```python
from build123d import *

# Parameters (mm, degrees)
SKETCH_W        = 40
SKETCH_H        = 26
PAD_DEPTH       = 6
SKETCH001_W     = 46
SKETCH001_H     = 21
POCKET_DEPTH    = 3.5
SKETCH002_R     = 1.7
POCKET001_DEPTH = 2.5
SKETCH003_W     = 20
SKETCH003_H     = 20
PAD001_DEPTH    = 15
SKETCH004_R     = 6.2
POCKET002_DEPTH = 15
FILLET_R        = 5


with BuildPart() as part:
    # Sketch → Pad (new body)
    with BuildSketch(Plane.XY):
        Rectangle(SKETCH_W, SKETCH_H)
    extrude(amount=PAD_DEPTH)

    # Sketch001 (on Face5 of Pad) → Pocket (cut)
    with BuildSketch(Plane(origin=(0, 0, 0), x_dir=(1, 0, 0), z_dir=(0, 0, -1))):
        Rectangle(SKETCH001_W, SKETCH001_H)
    extrude(amount=-POCKET_DEPTH, mode=Mode.SUBTRACT)

    # Sketch002 (on Face5 of Pocket) → Pocket001 (cut)
    with BuildSketch(Plane.XY.offset(6)):
        with Locations((-15, 5)):
            Circle(SKETCH002_R)
        with Locations((15, 5)):
            Circle(SKETCH002_R)
        with Locations((15, -5)):
            Circle(SKETCH002_R)
        with Locations((-15, -5)):
            Circle(SKETCH002_R)
    extrude(amount=-POCKET001_DEPTH, mode=Mode.SUBTRACT)

    # Sketch003 (on Face5 of Pocket001) → Pad001 (join)
    with BuildSketch(Plane.XY.offset(6)):
        Rectangle(SKETCH003_W, SKETCH003_H)
    extrude(amount=PAD001_DEPTH)

    # Sketch004 (on Face19 of Pad001) → Pocket002 (cut)
    with BuildSketch(Plane.XY.offset(21)):
        Circle(SKETCH004_R)
    extrude(amount=-POCKET002_DEPTH, mode=Mode.SUBTRACT)

    # Fillet
    fillet_edges = [part.edges().sort_by_distance(p)[0] for p in [
        (-10, -10, 13.5),
        (-10, 10, 13.5),
        (10, -10, 13.5),
        (10, 10, 13.5),
    ]]
    fillet(fillet_edges, radius=FILLET_R)


solid = part.part
```
Verification items for the finished model (mm, model axes). A direction names the side the tool comes from. Give positions to 0.01 mm unless a question says otherwise; leave off trailing zeros. Loops run counter-clockwise (first coordinate to the right, second up) from the corner with the lowest first, then second, coordinate; pieces in that order, holes last.
1. Section check B-B, the plane x = 15. Enter the section's corners in (y, z).
2. Section check A-A, the plane z = 19. Enter the section's corners in (x, y), then the cut area to 3 significant figures.
3. Mould release check, pull along X, two halves, no side actions. Record for faces 4 (the flat face through (20, 0, 4)), 5 (the flat face through (0, 0, 6)), 6 (the flat face through (-20, 0, 4)), 7 (the flat face through (0, -10, 13)): released by +X, released by -X, zero draft, split by the parting line, or undercut.
4. Thickness scan on line 1 (Y direction, x = 15, z = 4.4); line 2 (Y direction, x = 18.5, z = 2); line 3 (Z direction, x = 17.5, y = -6.75). Record the ranges inside material, lowest first.
5. Section check C-C, the plane y = 4.5. Enter the section's corners in (x, z), then the cut area to 3 significant figures.
6. Set-up check for faces 1 (the flat face through (0, 0, 3.5)), 2 (the flat face through (-10, 0, 13)), 3 (the flat face through (0, 10, 13)): record each of +Z, -Z, +X, -X, +Y, -Y from which the full face is reachable in a straight line by a thin tool's end or side.
7. Go/stop test with flat-tipped pins: pin 1 Ø5 at (x, z) = (-1, 13.5) entering from +Y; pin 2 Ø3.5 at (x, y) = (-2, 2.5) entering from +Z; pin 3 Ø10.5 at (x, y) = (4.5, 3) entering from -Z; pin 4 Ø2.5 at (x, y) = (-15, 5) entering from -Z. Record where each tip stops, or that it passes through.
8. Section check D-D, the plane z = 1.5. Enter the section's corners in (x, y), then the cut area to 3 significant figures.
Geometry says:
1. outline: (-13, 0) - (-10.5, 0) - (-10.5, 3.5) - (-6.7, 3.5) - (-6.7, 6) - (-13, 6) - close; (-3.3, 3.5) - (3.3, 3.5) - (3.3, 6) - (-3.3, 6) - close; (6.7, 3.5) - (10.5, 3.5) - (10.5, 0) - (13, 0) - (13, 6) - (6.7, 6) - close
2. outline: (-10, -5) arc R5 ccw to (-5, -10) - (5, -10) arc R5 ccw to (10, -5) - (10, 5) arc R5 ccw to (5, 10) - (-5, 10) arc R5 ccw to (-10, 5) - close; hole circle Ø12.4 at (0, 0)
2. area: 258 mm2
3. face 4: released by +X
3. face 5: undercut
3. face 6: released by -X
3. face 7: zero draft
4. line 1: y = -13 to -6.7, -3.3 to 3.3, 6.7 to 13
4. line 2: y = -13 to -10.5, 10.5 to 13
4. line 3: z = 3.5 to 6
5. outline: (-20, 3.5) - (-16.62, 3.5) - (-16.62, 6) - (-20, 6) - close; (-13.38, 3.5) - (13.38, 3.5) - (13.38, 6) - (10, 6) - (10, 21) - (4.26, 21) - (4.26, 6) - (-4.26, 6) - (-4.26, 21) - (-10, 21) - (-10, 6) - (-13.38, 6) - close; (16.62, 3.5) - (20, 3.5) - (20, 6) - (16.62, 6) - close
5. area: 256 mm2
6. face 1: -Z, +X, -X
6. face 2: +Z, -X, +Y, -Y
6. face 3: +Z, +X, -X, +Y
7. pin 1: stops at y = 10
7. pin 2: stops at z = 6
7. pin 3: stops at z = 3.5
7. pin 4: passes through
8. outline: (-20, -13) - (20, -13) - (20, -10.5) - (-20, -10.5) - close; (-20, 10.5) - (20, 10.5) - (20, 13) - (-20, 13) - close
8. area: 200 mm2
